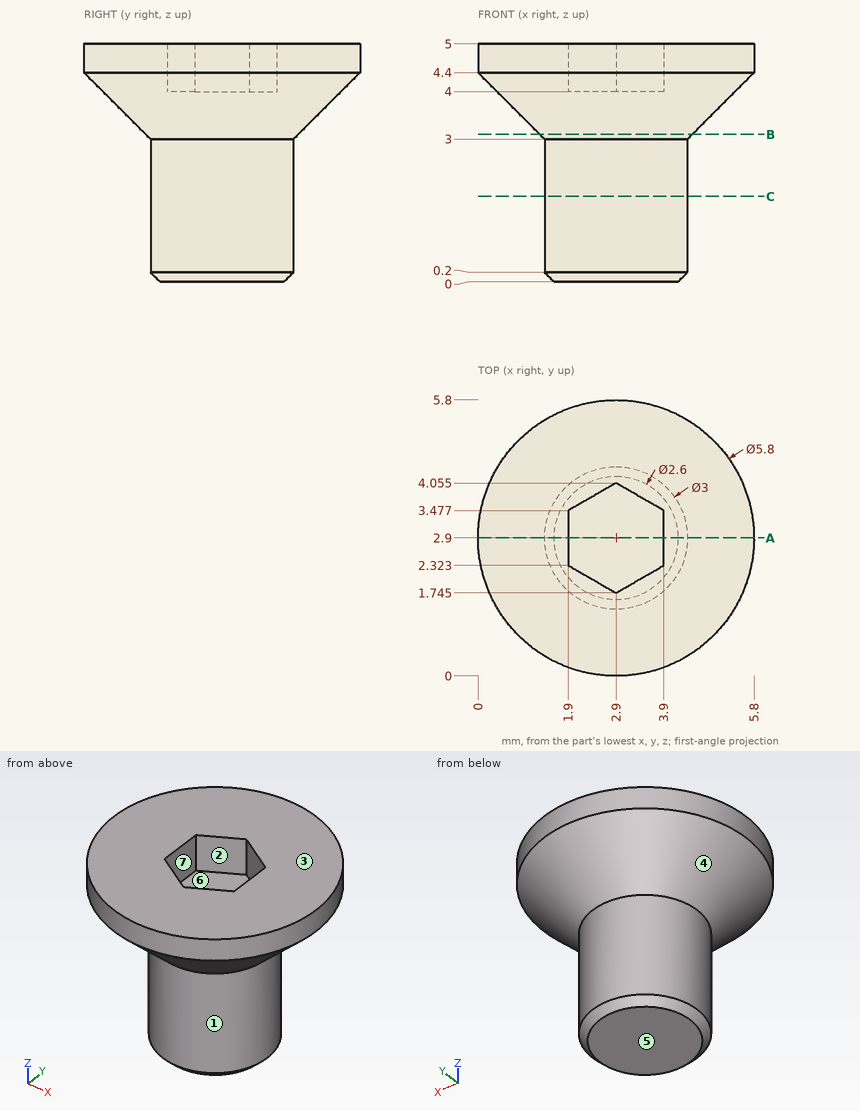
Here's the drawing with two shaded views (mm, measured from the low corner). I have some questions. A direction names the side the tool comes from. Coordinates: 2 decimals unless noted, no trailing zeros. Write each loop counter-clockwise with the first axis right and the second up, starting at its lowest first coordinate (ties: lowest second). Pieces come first, ordered by that corner, then holes. Notation, with made-up numbers: M 63,68 L 77,68 A29 ccw 77,106 Z; hole C -8.75,51 d7. An arc over 180 degrees is marked long. Answer as CSV lines item,"result". Start each with the question number.
1) For P1, Ø2, axis at x = 3, z = 2.5, coming from the -Y side; P2, Ø0.5, axis at y = 2.5, z = 4.5, coming from the +X side; P3, Ø1.6, axis at x = 3, y = 3.5, coming from the +Z side, each with a flat end and sliding along its axis, tell me the tip position at first contact or that it passes through.
2) For the marked faces 1, 2 and 3, which set-ups out of +Z, -Z, +X, -X, +Y, -Y let a thin tool reach every point of the face, with its end or its side?
3) Please list where these lines run through material, in increasing order: line 1 (Z direction, x = 3.55, y = 1); line 2 (Y direction, x = 2.8, z = 0.8); line 3 (Z direction, x = 0.9, y = 1.95) (1 decimal). Write a range as from..to.
4) I want a section at C-C, the plane z = 1.8. Please give me the cut outline in (x, y).
5) We'd pull the mould along Y, two halves only. Please class the marked faces 4, 5, 6 and 7: +Y half, -Y half, draft (parallel to the pull), parting line (faces both ways), or undercut.
6) I want a section at A-A, the plane y = 2.9. Please give me the cut outline in (x, z).
7) I want a section at B-B, the plane z = 3.1. Please give me the cut outline in (x, y).
Data:
1,P1,"stops at y = 0.9"
1,P2,"stops at x = 5.8"
1,P3,"stops at z = 5"
2,face 1,"-Z"
2,face 2,"+Z"
2,face 3,"+Z, +X, -X, +Y, -Y"
3,line 1,"z = 3.51..5"
3,line 2,"y = 1.4..4.4"
3,line 3,"z = 3.7..5"
4,outline,"C 2.9,2.9 d3"
5,face 4,"parting line"
5,face 5,"draft"
5,face 6,"undercut"
5,face 7,"undercut"
6,outline,"M 0,4.4 L 1.4,3 L 1.4,0.2 L 1.6,0 L 4.2,0 L 4.4,0.2 L 4.4,3 L 5.8,4.4 L 5.8,5 L 3.9,5 L 3.9,4 L 1.9,4 L 1.9,5 L 0,5 Z"
7,outline,"C 2.9,2.9 d3.2"
